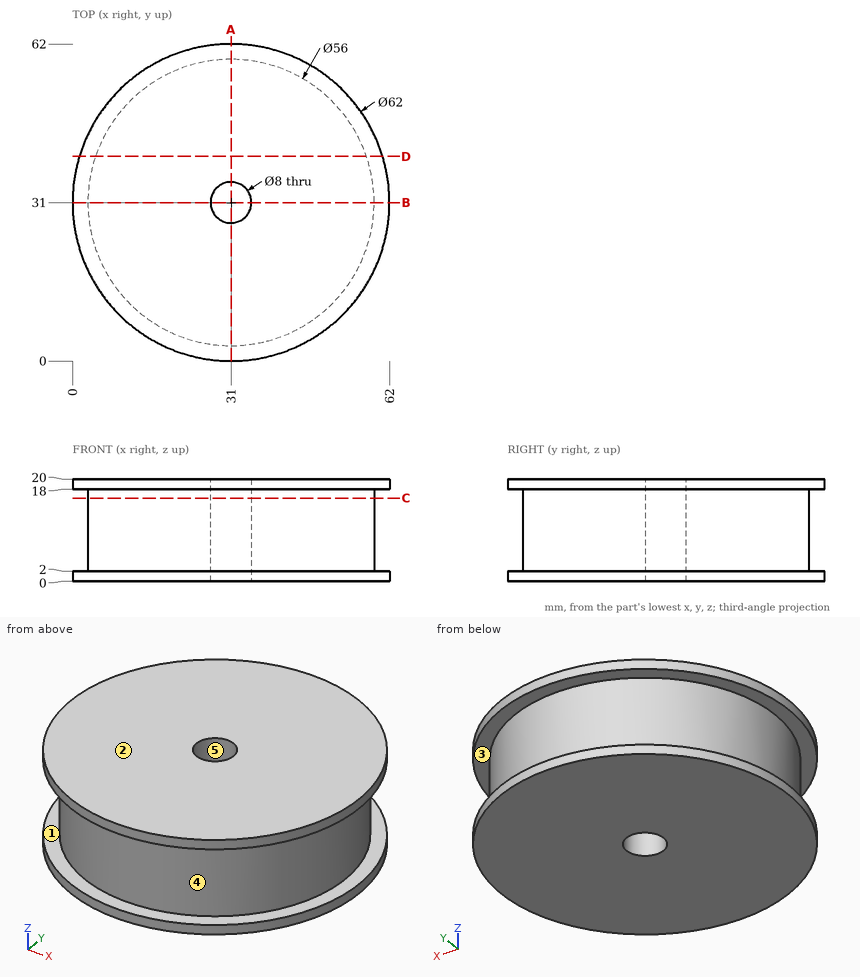
Verification items for this drawing (mm, ordinates from the low corner). A direction names the side the tool comes from. Coordinates: 2 decimals unless noted, no trailing zeros. Order: outer loops, then holes, each group sorted by start corner. A loop starts at its lowest first (then second) coordinate and runs counter-clockwise, first axis right, second up. Notation, with made-up numbers: (42, -7) - (55, -7) arc R19 cw to (55, 14) - close; hole circle Ø9 at (26, 41). An arc over 180 degrees is marked (long way). Answer in a Markdown table with one row per item. Add a question column.
1. Gauge pin test, flat ends, axial feed: pin 1 Ø2 at (x, z) = (34, 16) entering from +Y; pin 2 Ø2 at (x, y) = (23.5, 49) entering from -Z; pin 3 Ø12 at (y, z) = (32.5, 14) entering from -X; pin 4 Ø1.5 at (x, z) = (39.5, 11) entering from +Y. Record the tip position at first contact, or that the pin passes through.
2. Section check C-C (z = 16.25). Enter the section's corners in (x, y), plus the area to 3 significant figures.
3. Section check D-D (y = 40). Enter the section's corners in (x, z), plus the area to 3 significant figures.
4. Material ranges on L1, parallel to Y at x = 31, z = 4.25; L2, parallel to Z at x = 45, y = 57; L3, parallel to X at y = 32.5, z = 11.25, recorded low to high. Write a range as [from, to].
5. Section check A-A (x = 31). Enter the section's corners in (y, z), plus the area to 3 significant figures.
6. Access from +Z, -Z, +X, -X, +Y, -Y to the whole of each face (thin tool, end or side, straight path). Record for the marked faces 1 and 2.
7. Draft check along X on the marked faces 3, 4 and 5. Enter one of: +X half, -X half, draft (parallel to the pull), parting line (faces both ways), or undercut.
Data:
| question | item | result |
|---|---|---|
| 1 | pin 1 | stops at y = 58.93 |
| 1 | pin 2 | stops at z = 0 |
| 1 | pin 3 | stops at x = 0 |
| 1 | pin 4 | stops at y = 57.91 |
| 2 | outline | circle Ø56 at (31, 31); hole circle Ø8 at (31, 31) |
| 2 | area | 2,410 mm² |
| 3 | outline | (1.34, 0) - (60.66, 0) - (60.66, 2) - (57.51, 2) - (57.51, 18) - (60.66, 18) - (60.66, 20) - (1.34, 20) - (1.34, 18) - (4.49, 18) - (4.49, 2) - (1.34, 2) - close |
| 3 | area | 1,090 mm² |
| 4 | L1 | y = [3, 27], [35, 59] |
| 4 | L2 | z = [0, 2], [18, 20] |
| 4 | L3 | x = [3.04, 27.29], [34.71, 58.96] |
| 5 | outline | (0, 0) - (27, 0) - (27, 20) - (0, 20) - (0, 18) - (3, 18) - (3, 2) - (0, 2) - close; (35, 0) - (62, 0) - (62, 2) - (59, 2) - (59, 18) - (62, 18) - (62, 20) - (35, 20) - close |
| 5 | area | 984 mm² |
| 6 | face 1 | none |
| 6 | face 2 | +Z, +X, -X, +Y, -Y |
| 7 | face 3 | draft |
| 7 | face 4 | parting line |
| 7 | face 5 | undercut |
